For this review, use the dimensioned drawing (mm, ordinates from the lowest corner) and the shaded views. A direction names the side the tool comes from. Round coordinates to 2 decimals unless told otherwise and drop trailing zeros. Loops run counter-clockwise (first coordinate to the right, second up) from the corner with the lowest first, then second, coordinate; pieces in that order, holes last. Notation, with made-up numbers: (75.5, 84) -> (100.5, 84) arc R23 ccw to (100.5, 92) -> close; hole circle Ø7 at (45.25, 67). An arc over 180 degrees is marked (long way). Use one line per item in the form item = value. Start each with the question number.
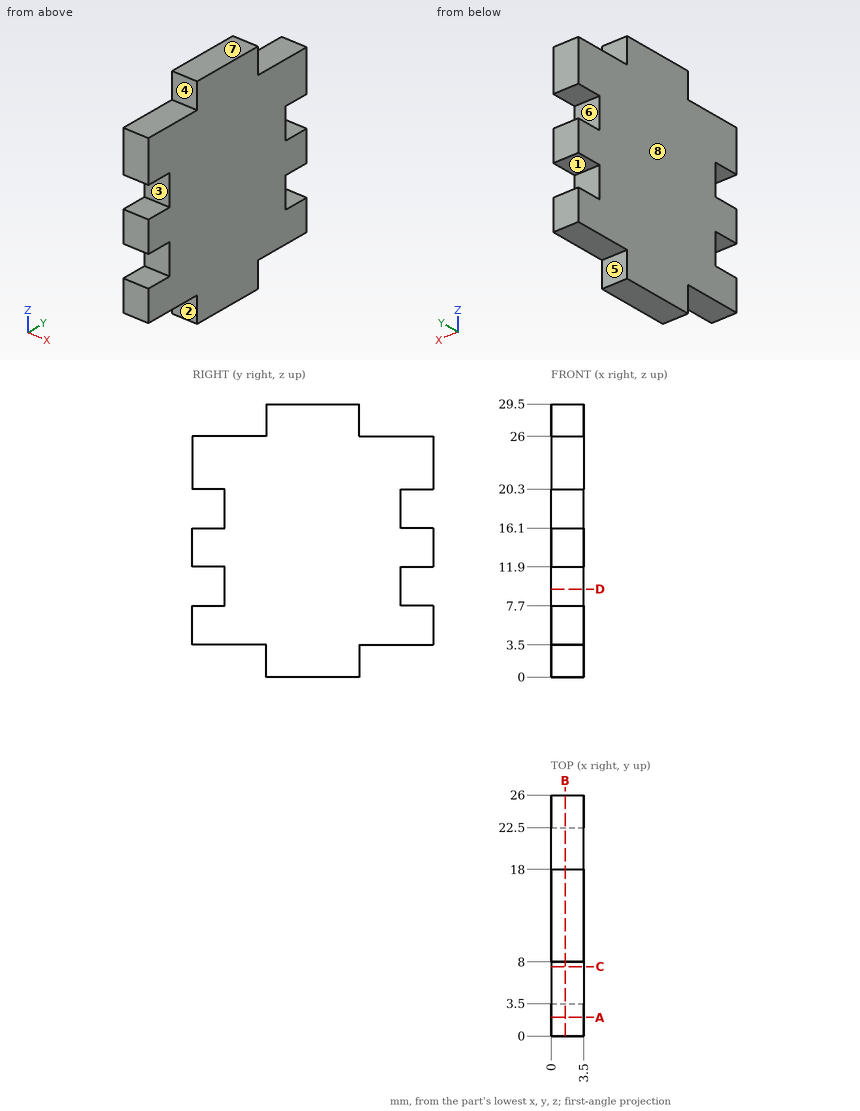
Item 1: Wall thickness on line 1 (Z direction, x = 2.9, y = 23.5); line 2 (Z direction, x = 2.35, y = 4.5); line 3 (Y direction, x = 0.35, z = 8.75): over which ranges is each line inside the solid? List them lowest first.
Item 2: Take a section at B-B on x = 1.5. Give the boundary of the cut face in (y, z), plus the area to 3 significant figures.
Item 3: For P1, Ø3, axis at y = 16.5, z = 17.5, coming from the -X side; P2, Ø1.8, axis at x = 2, y = 25, coming from the -Z side; P3, Ø1, axis at x = 2.5, z = 10.5, coming from the +Y side; P4, Ø1.8, axis at x = 1.5, y = 2, coming from the +Z side, all flat-tipped, find the tip position at first contact; note any pin that passes through.
Item 4: Take a section at A-A on y = 2. Give the boundary of the cut face in (x, z), plus the area to 4 significant figures.
Item 5: Take a section at D-D on z = 9.5. Give the boundary of the cut face in (x, y), plus the area to 3 significant figures.
Item 6: Machinability: for the marked faces 1, 2, 3, 4 and 5, which of the approach directions +Z, -Z, +X, -X, +Y, -Y give a long, thin tool a straight path to every point of the face, cutting with its end or side? Answer none if there is none.
Item 7: Draft analysis for pull direction Z (two halves, no side actions). For the marked faces 6, 7 and 8, state which applies: +Z half, -Z half, draft (parallel to the pull), parting line (faces both ways), or undercut.
Item 8: Take a section at C-C on y = 7.5. Give the boundary of the cut face in (x, z).
Results:
q1.line_1 = 3.5 to 7.7, 11.9 to 16.1, 20.3 to 26
q1.line_2 = 3.5 to 26
q1.line_3 = 3.5 to 22.5
q2.outline = (0, 3.5) -> (8, 3.5) -> (8, 0) -> (18, 0) -> (18, 3.5) -> (26, 3.5) -> (26, 7.7) -> (22.5, 7.7) -> (22.5, 11.9) -> (26, 11.9) -> (26, 16.1) -> (22.5, 16.1) -> (22.5, 20.3) -> (26, 20.3) -> (26, 26) -> (18, 26) -> (18, 29.5) -> (8, 29.5) -> (8, 26) -> (0, 26) -> (0, 20.3) -> (3.5, 20.3) -> (3.5, 16.1) -> (0, 16.1) -> (0, 11.9) -> (3.5, 11.9) -> (3.5, 7.7) -> (0, 7.7) -> close
q2.area = 596 mm2
q3.P1 = 0
q3.P2 = 3.5
q3.P3 = 22.5
q3.P4 = 26
q4.outline = (0, 3.5) -> (3.5, 3.5) -> (3.5, 7.7) -> (0, 7.7) -> close; (0, 11.9) -> (3.5, 11.9) -> (3.5, 16.1) -> (0, 16.1) -> close; (0, 20.3) -> (3.5, 20.3) -> (3.5, 26) -> (0, 26) -> close
q4.area = 49.35 mm2
q5.outline = (0, 3.5) -> (3.5, 3.5) -> (3.5, 22.5) -> (0, 22.5) -> close
q5.area = 66.5 mm2
q6.face_1 = +X, -X, +Y
q6.face_2 = -Z, +X, -X, -Y
q6.face_3 = +X, -X, -Y
q6.face_4 = +Z, +X, -X, -Y
q6.face_5 = -Z, +X, -X, +Y
q7.face_6 = undercut
q7.face_7 = +Z half
q7.face_8 = draft
q8.outline = (0, 3.5) -> (3.5, 3.5) -> (3.5, 26) -> (0, 26) -> close
